```python
from build123d import *

# Parameters (mm, degrees)
SKETCH2_W           = 60
SKETCH2_H           = 42.3
BOSS_EXTRUDE1_DEPTH = 13
SKETCH4_R           = 11
SKETCH4_R_2         = 2
CUT_EXTRUDE1_DEPTH  = 48.598760453
SKETCH5_R           = 4.015
CUT_EXTRUDE2_DEPTH  = 10
BOSS_EXTRUDE2_DEPTH = 53
CUT_EXTRUDE3_DEPTH  = 2.35
SKETCH8_R           = 1.5
CUT_EXTRUDE4_DEPTH  = 10


with BuildPart() as part:
    # Sketch2 → Boss-Extrude1 (new body)
    with BuildSketch(Plane.XY):
        with Locations((8.969325153, -2.892331288)):
            Rectangle(SKETCH2_W, SKETCH2_H)
    extrude(amount=-BOSS_EXTRUDE1_DEPTH)

    # Sketch4 → Cut-Extrude1 (cut, through all)
    with BuildSketch(Plane.XY):
        with Locations((8.969325153, -2.892331288)):
            Circle(SKETCH4_R)
        with Locations((24.469325153, 12.607668712)):
            Circle(SKETCH4_R_2)
        with Locations((-6.530674847, 12.607668712)):
            Circle(SKETCH4_R_2)
        with Locations((24.469325153, -18.392331288)):
            Circle(SKETCH4_R_2)
        with Locations((-6.530674847, -18.392331288)):
            Circle(SKETCH4_R_2)
    extrude(amount=-CUT_EXTRUDE1_DEPTH, mode=Mode.SUBTRACT)

    # Sketch5 → Cut-Extrude2 (cut)
    with BuildSketch(Plane.XY):
        with Locations((30.119325153, -2.892331288)):
            Circle(SKETCH5_R)
        with Locations(Location((-12.180674847, -2.892331288, 0), (0, 0, 180))):
            Circle(SKETCH5_R)
    extrude(amount=-CUT_EXTRUDE2_DEPTH, mode=Mode.SUBTRACT)

    # Sketch6 → Boss-Extrude2 (add)
    with BuildSketch(Plane.XY):
        Polygon((-21.030674847, 18.257668712), (-21.030674847, 43.257668712), (-13.530674847, 43.257668712), (8.969325153, 23.257668712), (31.469325153, 43.257668712), (38.969325153, 43.257668712), (38.969325153, 18.257668712), align=None)
    extrude(amount=-BOSS_EXTRUDE2_DEPTH)

    # Sketch7 → Cut-Extrude3 (cut)
    with BuildSketch(Plane(origin=(0, 43.257668712, 0), x_dir=(1, 0, 0), z_dir=(0, 1, 0))):
        Polygon((38.559325153, 10), (36.889325153, 12.892524849), (33.549325153, 12.892524849), (31.879325153, 10), (33.549325153, 7.107475151), (36.889325153, 7.107475151), align=None)
    extrude(amount=-CUT_EXTRUDE3_DEPTH, mode=Mode.SUBTRACT)

    # Sketch8 → Cut-Extrude4 (cut)
    with BuildSketch(Plane(origin=(0, 40.907668712, 0), x_dir=(1, 0, 0), z_dir=(0, 1, 0))):
        with Locations(Location((35.219325153, 10, 0), (0, 0, 270))):
            Circle(SKETCH8_R)
    extrude(amount=-CUT_EXTRUDE4_DEPTH, mode=Mode.SUBTRACT)


solid = part.part
```
Read the model definition and answer for the solid it produces. Units are mm, in the model's axes. A direction names the side the tool comes from. Coordinates: 2 decimals unless noted, no trailing zeros. Loops run counter-clockwise (first coordinate to the right, second up) from the corner with the lowest first, then second, coordinate; pieces in that order, holes last.
(1) Flat-ended cylindrical pins translate along their axes: pin 1 Ø8 at (x, z) = (4.5, -28.5) entering from +Y; pin 2 Ø6.5 at (x, y) = (24.47, -18.39) entering from -Z; pin 3 Ø3 at (x, y) = (14, 4) entering from -Z; pin 4 Ø2.5 at (x, z) = (35, -10.5) entering from +Y. Find the tip coordinate at first contact, or state that the pin passes through.
Solution:
pin 1: stops at y = 30.79
pin 2: stops at z = -13
pin 3: passes through
pin 4: stops at y = 40.91
(2) The part is cut by section A-A (y = -17.5). Determine the outline of the cut face in (x, z).
Solution:
outline: (-21.03, -13) - (-8.32, -13) - (-8.32, 0) - (-21.03, 0) - close; (-4.74, -13) - (22.68, -13) - (22.68, 0) - (-4.74, 0) - close; (26.26, -13) - (38.97, -13) - (38.97, 0) - (26.26, 0) - close
(3) A tool of negligible diameter and unlimited length cuts with its end or side. For faces 1 (the face through (37.71, 42.1, -8.53)), 2 (the face through (2, 7, -13)), 3 (the face through (22.995, -17.041, -6.409)), 4 (the face through (33.95, -1.69, -4.93)), 5 (the face through (-2.44, 33.4, -26.13)), from which of +Z, -Z, +X, -X, +Y, -Y can it reach the whole face along a straight path? Write none if from no direction.
Solution:
face 1: +Y
face 2: -Z, +X, -X, -Y
face 3: +Z, -Z
face 4: +Z
face 5: +Z, -Z, +Y
(4) The part is cut by section C-C (z = -32). Determine the outline of the cut face in (x, y).
Solution:
outline: (-21.03, 18.26) - (38.97, 18.26) - (38.97, 43.26) - (31.47, 43.26) - (8.97, 23.26) - (-13.53, 43.26) - (-21.03, 43.26) - close
(5) The mould has two halves that part along X. Classify faces 6 (the face through (35, 43.258, -26)), 7 (the face through (38.969, 25, -20)), 8 (the face through (35, 42, -12.893)): released by +X, released by -X, zero draft, split by the parting line, or undercut.
Solution:
face 6: zero draft
face 7: released by +X
face 8: undercut
(6) The part is cut by section D-D (y = -1). Determine the outline of the cut face in (x, z).
Solution:
outline: (-21.03, -13) - (-1.87, -13) - (-1.87, 0) - (-8.64, 0) - (-8.64, -10) - (-15.72, -10) - (-15.72, 0) - (-21.03, 0) - close; (19.81, -13) - (38.97, -13) - (38.97, 0) - (33.66, 0) - (33.66, -10) - (26.58, -10) - (26.58, 0) - (19.81, 0) - close
(7) The part is cut by section B-B (y = 36.5). Determine the outline of the cut face in (x, z), and give its area (3 significant figures).
Solution:
outline: (-21.03, -53) - (-5.93, -53) - (-5.93, 0) - (-21.03, 0) - close; (23.87, -53) - (38.97, -53) - (38.97, 0) - (23.87, 0) - close; hole circle Ø3 at (35.22, -10)
area: 1,590 mm2
(8) Consider line 1 along Y through (x, z) = (-7, -12); line 2 along Z through (x, y) = (-5, 15); line 3 along Y through (x, z) = (-8, -9). Determine where each line is inside the solid, lowest interval first.
Solution:
line 1: y = -24.04 to -20.34, -16.45 to 10.66, 14.55 to 37.45
line 2: z = -13 to 0
line 3: y = -24.04 to -19.75, -17.04 to 11.25, 13.96 to 38.34
